Read the model definition and answer for the solid it produces. Units are mm, in the model's axes. A direction names the side the tool comes from. Coordinates: 2 decimals unless noted, no trailing zeros. Write each loop counter-clockwise with the first axis right and the second up, starting at its lowest first coordinate (ties: lowest second). Pieces come first, ordered by that corner, then holes.
(1) Given pin 1 (3.5 mm diameter, centred on x = 49.39, z = 10, fed in from +Y); pin 2 (2 mm diameter, centred on y = 21.5, z = 3, fed in from +X); pin 3 (5.5 mm diameter, centred on x = -40.5, z = 15, fed in from +Y); pin 4 (2 mm diameter, centred on y = 12, z = 3.5, fed in from -X), each flat-ended and moving along its own axis, determine where each tip first touches the part or whether it passes through.
(2) The part is cut by section C-C, the plane y = 8. Determine the outline of the cut face in (x, z), and give its area (3 significant figures).
(3) Which of the six approach directions +Z, -Z, +X, -X, +Y, -Y give full straight-line access (tool end or side, diameter ignored) to faces 1 (the flat face through (53, 0, 10)), 2 (the flat face through (6, 32.3, 10)), 3 (the flat face through (-28.106, 18, 10))?
(4) Straight lines are drawn through the part: line 1 along X through (y, z) = (16.5, 10); line 2 along Y through (x, z) = (-14, 11.5); line 3 along Y through (x, z) = (-35, 13.75). For each, find the intervals that lie inside material, in ascending order.
(5) Determine the mould class of faces 4 (the cylindrical face through (-34.46, -2.53, 10.68)), 5 (the flat face through (56.894, -3, 10)), 6 (the flat face through (-44.106, -2, 10)) for opening direction X: pulls with the +X half, pulls with the -X half, needs draft (parallel to the pull), parting line crosses it, or undercut.
(6) The part is cut by section A-A, the plane y = -1. Determine the outline of the cut face in (x, z), and give its area (3 significant figures).
(7) The part is cut by section D-D, the plane x = 24. Determine the outline of the cut face in (y, z).
(8) The part is cut by section B-B, the plane z = 10. Determine the outline of the cut face in (x, y).
```python
from build123d import *

# Parameters (mm, degrees)
F0_W     = 61
F0_H     = 3
F0_W_2   = 4
F0_H_2   = 32.3
F1_DEPTH = 20
F2_R     = 5
F5_D     = 4.5
F6_R     = 5
F7_R     = 5
F8_R     = 5


with BuildPart() as f1:
    # F0 (on Top) → F1 (new body)
    with BuildSketch(Plane.XY):
        Polygon((-28.105963, 0), (-44.105963, 0), (-44.105963, -5), (-24.105963, -5), (-24.105963, 0), align=None)
        Polygon((-28.105963, 35.3), (-28.105963, 0), (-24.105963, 0), (-24.105963, 32.3), (-24.105963, 35.3), align=None)
        with Locations((6.394037, 33.8)):
            Rectangle(F0_W, F0_H)
        with Locations((38.894037, 33.8)):
            Rectangle(F0_W_2, F0_H)
        with Locations((38.894037, 16.15)):
            Rectangle(F0_W_2, F0_H_2)
        Polygon((40.894037, 0), (36.894037, 0), (36.894037, -5), (56.894037, -5), (56.894037, 0), align=None)
    extrude(amount=F1_DEPTH)

    # F2
    f2_edges = [f1.edges().sort_by_distance(p)[0] for p in [
        (-24.105963, 32.3, 10),
        (36.894037, 32.3, 10),
    ]]
    fillet(f2_edges, radius=F2_R)

    # F5 (through all)
    with Locations(Plane(origin=(0, 0, 0), x_dir=(-1, 0, 0), z_dir=(0, 1, 0))):
        with Locations((36.605963, 10), (-49.394037, 10)):
            Hole(F5_D / 2)

    # F6
    f6_edges = [f1.edges().sort_by_distance(p)[0] for p in [
        (-28.105963, 35.3, 10),
        (40.894037, 35.3, 10),
    ]]
    fillet(f6_edges, radius=F6_R)

    # F7
    f7_edges = [f1.edges().sort_by_distance(p)[0] for p in [
        (-28.105963, 0, 10),
        (40.894037, 0, 10),
    ]]
    fillet(f7_edges, radius=F7_R)

    # F8
    f8_edges = [f1.edges().sort_by_distance(p)[0] for p in [
        (56.894037, -2.5, 20),
        (56.894037, -2.5, 0),
        (-44.105963, -2.5, 0),
        (-44.105963, -2.5, 20),
    ]]
    fillet(f8_edges, radius=F8_R)


solid = f1.part
```
Computed:
1. pin 1: passes through
1. pin 2: stops at x = 40.89
1. pin 3: stops at y = 0
1. pin 4: stops at x = -28.11
2. outline: (-28.11, 0) - (-24.11, 0) - (-24.11, 20) - (-28.11, 20) - close; (36.89, 0) - (40.89, 0) - (40.89, 20) - (36.89, 20) - close
2. area: 160 mm2
3. face 1: +Z, -Z, +X, +Y
3. face 2: +Z, -Z, -Y
3. face 3: +Z, -Z, -X, +Y
4. line 1: x = -28.11 to -24.11, 36.89 to 40.89
4. line 2: y = 32.3 to 35.3
4. line 3: y = -5 to 0
5. face 4: undercut
5. face 5: pulls with the +X half
5. face 6: pulls with the -X half
6. outline: (-44.11, 5) arc R5 ccw to (-39.11, 0) - (-24.11, 0) - (-24.11, 20) - (-39.11, 20) arc R5 ccw to (-44.11, 15) - close; (36.89, 0) - (51.89, 0) arc R5 ccw to (56.89, 5) - (56.89, 15) arc R5 ccw to (51.89, 20) - (36.89, 20) - close; hole circle Ø4.5 at (-36.61, 10); hole circle Ø4.5 at (49.39, 10)
6. area: 747 mm2
7. outline: (32.3, 0) - (35.3, 0) - (35.3, 20) - (32.3, 20) - close
8. outline: (-44.11, -5) - (-38.86, -5) - (-38.86, 0) - (-44.11, 0) - close; (-34.36, -5) - (-24.11, -5) - (-24.11, 27.3) arc R5 cw to (-19.11, 32.3) - (31.89, 32.3) arc R5 cw to (36.89, 27.3) - (36.89, -5) - (47.14, -5) - (47.14, 0) - (45.89, 0) arc R5 cw to (40.89, 5) - (40.89, 30.3) arc R5 ccw to (35.89, 35.3) - (-23.11, 35.3) arc R5 ccw to (-28.11, 30.3) - (-28.11, 5) arc R5 cw to (-33.11, 0) - (-34.36, 0) - close; (51.64, -5) - (56.89, -5) - (56.89, 0) - (51.64, 0) - close
